```python
from build123d import *

# Parameters (mm, degrees)
SKETCH1_W               = 412.75
SKETCH1_H               = 403.225
BOSS_EXTRUDE1_DEPTH     = 3.175
SKETCH2_W               = 3.175
SKETCH2_H               = 87.3125
CUT_EXTRUDE1_DEPTH      = 3.175
SKETCH3_W               = 3.175
SKETCH3_H               = 12.7
CUT_EXTRUDE2_DEPTH      = 3.175
SKETCH4_W               = 3.175
SKETCH4_H               = 12.7
CUT_EXTRUDE3_DEPTH      = 3.175
MIRROR2_COPY_1_SKETCH_W = 3.175
MIRROR2_COPY_1_SKETCH_H = 12.7
MIRROR2_COPY_1_DEPTH    = 3.175
CUT_EXTRUDE4_DEPTH      = 3.175
MIRROR4_COPY_1_DEPTH    = 3.175


with BuildPart() as part:
    # Sketch1 → Boss-Extrude1 (new body)
    with BuildSketch(Plane(origin=(0, 0, 0), x_dir=(1, 0, 0), z_dir=(0, 1, 0))):
        Rectangle(SKETCH1_W, SKETCH1_H)
    extrude(amount=BOSS_EXTRUDE1_DEPTH)

    # Sketch2 → Cut-Extrude1 (cut)
    with BuildSketch(Plane(origin=(0, 3.175, 0), x_dir=(1, 0, 0), z_dir=(0, 1, 0))):
        with Locations((-204.7875, 81.75625)):
            Rectangle(SKETCH2_W, SKETCH2_H)
        with Locations((-204.7875, -81.75625)):
            Rectangle(SKETCH2_W, SKETCH2_H)
    cut_extrude1 = extrude(amount=-CUT_EXTRUDE1_DEPTH, mode=Mode.SUBTRACT)

    # Sketch3 → Cut-Extrude2 (cut)
    with BuildSketch(Plane(origin=(0, 3.175, 0), x_dir=(1, 0, 0), z_dir=(0, 1, 0))):
        with Locations((-204.7875, 201.6125)):
            Rectangle(SKETCH3_W, SKETCH3_H)
        with Locations((-204.7875, 176.2125)):
            Rectangle(SKETCH3_W, SKETCH3_H)
        with Locations((-204.7875, 150.8125)):
            Rectangle(SKETCH3_W, SKETCH3_H)
        with Locations((-204.7875, 125.4125)):
            Rectangle(SKETCH3_W, SKETCH3_H)
    cut_extrude2 = extrude(amount=-CUT_EXTRUDE2_DEPTH, mode=Mode.SUBTRACT)

    # Sketch4 → Cut-Extrude3 (cut)
    with BuildSketch(Plane(origin=(0, 3.175, 0), x_dir=(1, 0, 0), z_dir=(0, 1, 0))):
        with Locations((-204.7875, 38.1)):
            Rectangle(SKETCH4_W, SKETCH4_H)
        with Locations((-204.7875, 12.7)):
            Rectangle(SKETCH4_W, SKETCH4_H)
        with Locations((-204.7875, -12.7)):
            Rectangle(SKETCH4_W, SKETCH4_H)
        with Locations((-204.7875, -38.1)):
            Rectangle(SKETCH4_W, SKETCH4_H)
    cut_extrude3 = extrude(amount=-CUT_EXTRUDE3_DEPTH, mode=Mode.SUBTRACT)

    # Mirror1: Cut-Extrude2 across plane
    add(cut_extrude2.mirror(Plane.XY), mode=Mode.SUBTRACT)

    # Mirror2: Cut-Extrude1, Cut-Extrude2, Cut-Extrude3 across plane
    add(cut_extrude1.mirror(Plane(origin=(0, 0, 0), x_dir=(0, 0, 1), z_dir=(1, 0, 0))), mode=Mode.SUBTRACT)
    add(cut_extrude2.mirror(Plane(origin=(0, 0, 0), x_dir=(0, 0, 1), z_dir=(1, 0, 0))), mode=Mode.SUBTRACT)
    add(cut_extrude3.mirror(Plane(origin=(0, 0, 0), x_dir=(0, 0, 1), z_dir=(1, 0, 0))), mode=Mode.SUBTRACT)

    # Mirror2 copy 1 sketch → Mirror2 copy 1 (cut)
    with BuildSketch(Plane(origin=(0, 3.175, 0), x_dir=(-1, 0, 0), z_dir=(0, 1, 0))):
        with Locations((-204.7875, 201.6125)):
            Rectangle(MIRROR2_COPY_1_SKETCH_W, MIRROR2_COPY_1_SKETCH_H)
        with Locations((-204.7875, 176.2125)):
            Rectangle(MIRROR2_COPY_1_SKETCH_W, MIRROR2_COPY_1_SKETCH_H)
        with Locations((-204.7875, 150.8125)):
            Rectangle(MIRROR2_COPY_1_SKETCH_W, MIRROR2_COPY_1_SKETCH_H)
        with Locations((-204.7875, 125.4125)):
            Rectangle(MIRROR2_COPY_1_SKETCH_W, MIRROR2_COPY_1_SKETCH_H)
    extrude(amount=-MIRROR2_COPY_1_DEPTH, mode=Mode.SUBTRACT)

    # Sketch5 → Cut-Extrude4 (cut)
    with BuildSketch(Plane(origin=(0, 3.175, 0), x_dir=(1, 0, 0), z_dir=(0, 1, 0))):
        Polygon((-190.5, 6.35), (-36.183770369, 6.35), (-189.462331729, 69.064060773), (-189.581560693, 82.834747968), (-24.310343952, 15.213881497), (-190.5, 179.970868096), align=None)
        Polygon((-181.480614775, 188.9125), (-15.369047179, 24.232928676), (-84.41827204, 188.9125), align=None)
        Polygon((-70.647068702, 188.9125), (-6.35, 35.566626349), (-6.35, 188.9125), align=None)
    cut_extrude4 = extrude(amount=-CUT_EXTRUDE4_DEPTH, mode=Mode.SUBTRACT)

    # Mirror3: Cut-Extrude4 across plane
    add(cut_extrude4.mirror(Plane(origin=(0, 0, 0), x_dir=(0, 0, 1), z_dir=(1, 0, 0))), mode=Mode.SUBTRACT)

    # Mirror4: Cut-Extrude4 across plane
    add(cut_extrude4.mirror(Plane.XY), mode=Mode.SUBTRACT)

    # Mirror4 copy 1 sketch → Mirror4 copy 1 (cut)
    with BuildSketch(Plane(origin=(0, 3.175, 0), x_dir=(-1, 0, 0), z_dir=(0, 1, 0))):
        Polygon((-190.5, 6.35), (-36.183770369, 6.35), (-189.462331729, 69.064060773), (-189.581560693, 82.834747968), (-24.310343952, 15.213881497), (-190.5, 179.970868096), align=None)
        Polygon((-181.480614775, 188.9125), (-15.369047179, 24.232928676), (-84.41827204, 188.9125), align=None)
        Polygon((-70.647068702, 188.9125), (-6.35, 35.566626349), (-6.35, 188.9125), align=None)
    extrude(amount=-MIRROR4_COPY_1_DEPTH, mode=Mode.SUBTRACT)


solid = part.part
```
Geometry: final body of the model. Coordinates: model frame, mm. Coordinates: 2 decimals unless noted, no trailing zeros. Loops run counter-clockwise (first coordinate to the right, second up) from the corner with the lowest first, then second, coordinate; pieces in that order, holes last. Notation, with made-up numbers: M 22.25,60.25 L 28.25,60.25 A9 cw 28.25,66.25 Z; hole C 87.5,29.25 d7. An arc over 180 degrees is marked long. Put each result on its own line as item: value.
(1) Cut plane B-B on z = 138. Return the cut outline in (x, y) (3 decimals), then the cut area to 3 significant figures.
Answer sheet:
outline: M -206.375,0 L -190.5,0 L -190.5,3.175 L -206.375,3.175 Z; M -148.164,0 L -130.125,0 L -130.125,3.175 L -148.164,3.175 Z; M -63.071,0 L -49.3,0 L -49.3,3.175 L -63.071,3.175 Z; M -6.35,0 L 6.35,0 L 6.35,3.175 L -6.35,3.175 Z; M 49.3,0 L 63.071,0 L 63.071,3.175 L 49.3,3.175 Z; M 130.125,0 L 148.164,0 L 148.164,3.175 L 130.125,3.175 Z; M 190.5,0 L 206.375,0 L 206.375,3.175 L 190.5,3.175 Z
area: 343 mm^2
(2) Draft query along Z for faces 1 (the face through (111.75, 1.61, -37.27)), 2 (the face through (-3, 3.175, -3)). Return one class per face: pulls with the +Z half, pulls with the -Z half, needs draft (parallel to the pull), parting line crosses it, or undercut.
Answer sheet:
face 1: undercut
face 2: needs draft
(3) First-contact query: pin 1 (1 mm diameter, centred on x = -205, y = 1.5, fed in from -Z); pin 2 (1.6 mm diameter, centred on y = 1.5, z = 150, fed in from -X); pin 3 (1 mm diameter, centred on y = 2.5, z = -145, fed in from +X). Flat tips, straight axial feed; report the tip coordinate or a pass-through.
Answer sheet:
pin 1: stops at z = -195.26
pin 2: stops at x = -203.2
pin 3: stops at x = 203.2
(4) Material intervals for probe 1 along X at (y, z) = (1.7, -8), sorted ascending.
Answer sheet:
probe 1: x = -203.2 to -190.5, -40.22 to 40.22, 190.5 to 203.2
(5) Cut plane A-A on x = -147. State how many separate pieces and enclosed holes the cut face has, then the cut area to 3 significant figures.
Answer sheet:
separate pieces: 7
enclosed holes: 0
area: 322 mm^2
